For this review, take the finished solid that the model builds, in its own axes (mm). A direction names the side the tool comes from. Coordinates: 2 decimals unless noted, no trailing zeros. Order: outer loops, then holes, each group sorted by start corner. A loop starts at its lowest first (then second) coordinate and runs counter-clockwise, first axis right, second up. Notation, with made-up numbers: M 82.25,-27.75 L 124.25,-27.75 A21 cw 124.25,-2.75 Z; hole C 84,62.5 d4. An arc over 180 degrees is marked long. Use CSV: the item, a comma, the result in double quotes.
```python
from build123d import *

# Parameters (mm, degrees)
SKETCH1_W                 = 225.11
SKETCH1_H                 = 61.32
BOSS_EXTRUDE1_DEPTH       = 5
SKETCH2_R                 = 2.1
SKETCH2_W                 = 40
SKETCH2_H                 = 5
CUT_EXTRUDE1_DEPTH        = 5
BOSS_EXTRUDE2_START       = -5
BOSS_EXTRUDE2_DEPTH       = 5
BOSS_EXTRUDE2_2_OUTLINE_W = 40
BOSS_EXTRUDE2_2_OUTLINE_H = 5
BOSS_EXTRUDE2_2_DEPTH     = 5


# Read off the part's stored shape, not the designer's step: Boss-Extrude2
with BuildPart() as part:
    # Sketch1 → Boss-Extrude1 (new body)
    with BuildSketch(Plane.XY):
        Rectangle(SKETCH1_W, SKETCH1_H)
    extrude(amount=BOSS_EXTRUDE1_DEPTH)

    # Sketch2 → Cut-Extrude1 (cut)
    with BuildSketch(Plane.XY.offset(5)):
        with Locations((0.014505864, -4.956)):
            Circle(SKETCH2_R)
        with Locations((52.569505864, -4.956)):
            Rectangle(SKETCH2_W, SKETCH2_H)
        with Locations((-52.540494136, -4.956)):
            Rectangle(SKETCH2_W, SKETCH2_H)
    extrude(amount=-CUT_EXTRUDE1_DEPTH, mode=Mode.SUBTRACT)

    # Boss-Extrude2 outline → Boss-Extrude2 (cut)
    with BuildSketch(Plane.XY.offset(5).offset(BOSS_EXTRUDE2_START)):
        Polygon((109.555, -2.456), (109.555, -1.056), (112.555, -1.056), (112.555, 3.144), (109.555, 3.144), (109.555, 4.544), (106.755, 4.544), (106.755, 3.144), (95.555, 3.144), (95.555, -1.056), (106.755, -1.056), (106.755, -2.456), align=None)
        Polygon((-112.555, 3.144), (-112.555, -1.056), (-109.555, -1.056), (-109.555, -2.456), (-106.755, -2.456), (-106.755, -1.056), (-95.555, -1.056), (-95.555, 3.144), (-106.755, 3.144), (-106.755, 4.544), (-109.555, 4.544), (-109.555, 3.144), align=None)
    extrude(amount=BOSS_EXTRUDE2_DEPTH, mode=Mode.SUBTRACT)

    # Boss-Extrude2 2 outline → Boss-Extrude2 2 (add)
    with BuildSketch(Plane.XY.offset(5).offset(BOSS_EXTRUDE2_START)):
        with Locations((0, -33.16)):
            Rectangle(BOSS_EXTRUDE2_2_OUTLINE_W, BOSS_EXTRUDE2_2_OUTLINE_H)
    extrude(amount=BOSS_EXTRUDE2_2_DEPTH)


solid = part.part
```
Item 1: Add section B-B on x = 78. State the section outline as (y, z) points, and give its area (3 significant figures).
Solutions:
outline,"M -30.66,0 L 30.66,0 L 30.66,5 L -30.66,5 Z"
area,"307 mm^2"
Item 2: For faces 1 (the face through (95.555, 1, 2)), 2 (the face through (-72.54, -5, 3)), 3 (the face through (-67, -30.66, 2)), list the 3-axis set-ups (+Z, -Z, +X, -X, +Y, -Y) from which the entire face can be reached by the end or side of a thin tool; tool diameter is ignored.
Solutions:
face 1,"+Z, -Z, +X"
face 2,"+Z, -Z"
face 3,"+Z, -Z, -X, -Y"
Item 3: To check wall thickness, follow line 1 along X through (y, z) = (4, 3.8) (3 decimals); line 2 along Y through (x, z) = (61, 3.9); line 3 along Y through (x, z) = (-99, 2.55). State the ranges of each line that lie inside material, in increasing order. Write a range as [from, to].
Solutions:
line 1,"[-112.555, -109.555], [-106.755, 106.755], [109.555, 112.555]"
line 2,"[-30.66, -7.46], [-2.46, 30.66]"
line 3,"[-30.66, -1.06], [3.14, 30.66]"
Item 4: Add section C-C on z = 3. State how many separate pieces and enclosed holes the cut face has, and give its area (3 significant figures).
Solutions:
separate pieces,"1"
enclosed holes,"3"
area,"13,400 mm^2"
Item 5: Add section A-A on x = -37.5. State the section outline as (y, z) points.
Solutions:
outline,"M -30.66,0 L -7.46,0 L -7.46,5 L -30.66,5 Z; M -2.46,0 L 30.66,0 L 30.66,5 L -2.46,5 Z"
Item 6: Clearance check with flat-ended pins moving along their axes: pin 1 Ø2 at (x, z) = (-108, 3) entering from -Y; pin 2 Ø8 at (x, y) = (-10, 11.5) entering from -Z; pin 3 Ø1.5 at (y, z) = (-33.5, 1.5) entering from -X. State where each tip first meets the part, or that it passes through.
Solutions:
pin 1,"y = -30.66"
pin 2,"z = 0"
pin 3,"x = -20"
Item 7: Draft analysis for pull direction X (two halves, no side actions). For faces 4 (the face through (-2.083, -4.864, 2.535)), 5 (the face through (112.555, -16, 2)), 6 (the face through (72.57, -5, 3)), 7 (the face through (-20, -33, 2)), state which applies: released by +X, released by -X, zero draft, split by the parting line, or undercut.
Solutions:
face 4,"undercut"
face 5,"released by +X"
face 6,"undercut"
face 7,"released by -X"
